Work out the finished part from the listing and answer in its coordinate system (mm). Face numbers are marked on the shaded views. A direction names the side the tool comes from. Round coordinates to 2 decimals unless told otherwise and drop trailing zeros. Write each loop counter-clockwise with the first axis right and the second up, starting at its lowest first coordinate (ties: lowest second). Pieces come first, ordered by that corner, then holes. Notation, with made-up numbers: (39.25, -30.5) - (52.25, -30.5) arc R21 ccw to (52.25, -17.5) - close; hole circle Ø8 at (75, -6.75). An arc over 180 degrees is marked (long way). Write item = value, one per line. Start each with the question number.
Autodesk Inventor part; units mm, degrees
ref_plane "Work Plane1" through (127.7, -30, -88) normal (0, 0, -1) x (-1, 0, 0)
ref_plane "YZ Plane" through (0, 0, 0) normal (1, 0, 0) x (0, 1, 0)
ref_plane "XZ Plane" through (0, 0, 0) normal (0, 1, 0) x (-1, 0, 0)
sketch "Sketch1" plane through (0, 0, 0) normal (0, 0, 1) x (1, 0, 0)
  line L0 (-36, 36) -> (36, 36)
  line L1 (36, 36) -> (36, -36)
  line L2 (36, -36) -> (-36, -36)
  line L3 (-36, -36) -> (-36, 36)
  point P0 (0, 0)
  dimension "d0" = 72
  dimension "d1" = 36
  dimension "d2" = 72
  dimension "d3" = 36
extrude "Plate1" add sketch "Sketch1" along normal blind 6
sketch "Sketch2" plane through (-36, -30, 6) normal (0, -1, 0) x (1, 0, 0)
  line L0 (72, 0) -> (0, 0)
  line L1 (0, 0) -> (0, -94)
  line L2 (0, -94) -> (72, -94)
  line L3 (72, -94) -> (72, 0)
edge flange "Flange1" height 94 angle 90 thickness 6 bend radius 6 thickness toward (0, -1, 0) relief tear relief width 6 relief depth 3 edges at (0, -36, 0) wall of the first edge with corners at (36, -30, 6) (-36, -30, 6) (-36, -30, -88) (36, -30, -88)
bend "Bend1"
corner "Corner1"
sketch "Sketch3" plane through (-36, -30, -88) normal (0, 1, 0) x (1, 0, 0)
  line L0 (72, -82) -> (72, 0)
  line L1 (72, 0) -> (175.7, 0)
  line L2 (175.7, 0) -> (175.7, -60)
  line L3 (175.7, -60) -> (72, -60)
  line L4 (72, -60) -> (72, 0)
  point P0 (36, -88)
  dimension "d15" = 103.7
  dimension "d16" = 60
sheet face with bend "Face2" sketch "Sketch3" thickness 6 toward (0, -1, 0) bend radius 6
bend "Bend2"
sketch "Sketch4" plane through (133.7, -36, -88) normal (1, 0, 0) x (0, 1, 0)
  line L0 (0, 60) -> (0, 0)
  line L1 (0, 0) -> (100.6, 0)
  line L2 (100.6, 0) -> (100.6, 60)
  line L3 (100.6, 60) -> (0, 60)
edge flange "Flange2" height 100.6 angle 90 thickness 6 bend radius 6 thickness toward (1, 0, 0) relief tear relief width 6 relief depth 3 edges at (139.7, -30, -58) wall of the first edge with corners at (133.7, -36, -28) (133.7, -36, -88) (133.7, 64.6, -88) (133.7, 64.6, -28)
bend "Bend3"
corner "Corner2"
sketch "Sketch5" plane through (139.7, 64.6, -28) normal (1, 0, 0) x (0, 0, -1)
  circle A0 centre (30, -30) radius 25
  line L0 (60, 0) -> (60, -88.6)
  line L1 (0, -88.6) -> (0, 0)
  line L2 (0, 0) -> (60, 0)
  point P0 (-28, -64.6)
  point P1 (55, -30)
  point P2 (5, -30)
  dimension "d32" = 60
  dimension "d33" = 30
  dimension "d34" = 30
  dimension "d35" = 50
  dimension "d36" = 30
  dimension "d37" = 30
hole "Hole1" at (139.7, 34.6, -33) at (139.7, 34.6, -83) direction (-1, 0, 0) diameter 5 end through all
sketch "Sketch6" plane through (0, 0, 6) normal (0, 0, 1) x (1, 0, 0)
  circle A0 centre (0, 0) radius 12.7
  line L0 (36, -36) -> (-36, -36)
  circle A1 centre (0, 0) radius 33.5
  line L1 (0, 0) -> (29.0119, -16.75)
  line L2 (0, 0) -> (-29.0119, -16.75)
  line L3 (0, 0) -> (0, 33.5)
  point P0 (0, 0)
  point P1 (0, 12.7)
  point P2 (10.9985, -6.35)
  point P3 (-10.9985, -6.35)
  dimension "d45" = 36
  dimension "d46" = 25.4
  dimension "d47" = 67
  dimension "d48" = 120
  dimension "d49" = 120
  dimension "d50" = 0
hole "Hole2" at (0, 12.7, 6) at (-10.9985, -6.35, 6) at (10.9985, -6.35, 6) at (29.0119, -16.75, 6) at (-29.0119, -16.75, 6) direction (0, 0, -1) diameter 5 end through all
sketch "Sketch7" plane through (-36, -30, -6) normal (0, 1, 0) x (1, 0, 0)
  line L0 (163.7, 82) -> (0, 82)
  line L1 (163.7, 22) -> (72, 22)
  line L2 (0, 0) -> (0, 82)
  line L3 (72, 0) -> (72, 22)
  point P0 (36, -6)
  point P1 (117.85, 52)
  point P2 (36, 52)
  point P3 (36, 11)
  dimension "d65" = 60
  dimension "d66" = 72
  dimension "d67" = 30
  dimension "d68" = 30
  dimension "d69" = 36
  dimension "d70" = 22
  dimension "d71" = 11
  dimension "d72" = 36
  dimension "d73" = 91.7
  dimension "d74" = 45.85
hole "Hole3" at (81.85, -30, -58) at (0, -30, -58) at (0, -30, -17) direction (0, -1, 0) diameter 5 end through all
mirror "Mirror1" about plane through (133.7, -24, -88) normal (0, 0, -1)
ref_plane "Work Plane1" through (127.7, -30, -88) normal (0, 0, -1) x (-1, 0, 0)
split "Split1" plane through (127.7, -30, -88) removes the side toward (0, 0, 1)
equation "\"d2\" = d0"
equation "\"d33\" = 0.5 * d32"
equation "\"d34\" = d33"
equation "\"d36\" = d34"
equation "\"d37\" = d36"
equation "\"d43\" = Thickness"
equation "\"d49\" = d48"
equation "\"d56\" = Thickness"
equation "\"d63\" = Thickness"
equation "\"d4\" = Thickness"
equation "\"d5\" = BendReliefWidth"
equation "\"d6\" = BendReliefDepth"
equation "\"d7\" = MinimumRemnant"
equation "\"d8\" = TransitionRadius"
equation "\"d11\" = BendRadius"
equation "\"d12\" = CornerReliefSize"
equation "\"d13\" = GapSize"
equation "\"d14\" = JacobiRadiusSize"
equation "\"d17\" = BendRadius"
equation "\"d18\" = BendReliefWidth"
equation "\"d20\" = MinimumRemnant"
equation "\"d19\" = BendReliefDepth"
equation "\"d21\" = TransitionRadius"
equation "\"d22\" = BendReliefWidth"
equation "\"d23\" = BendReliefDepth"
equation "\"d24\" = MinimumRemnant"
equation "\"d25\" = TransitionRadius"
equation "\"d28\" = BendRadius"
equation "\"d29\" = CornerReliefSize"
equation "\"d30\" = GapSize"
equation "\"d31\" = JacobiRadiusSize"
equation "\"BendRadius\" = Thickness"
equation "\"BendReliefWidth\" = Thickness"
equation "\"BendReliefDepth\" = 0.5 * Thickness"
equation "\"CornerReliefSize\" = 4 * Thickness"
equation "\"MinimumRemnant\" = 2 * Thickness"
equation "\"TransitionRadius\" = BendRadius"
equation "\"JacobiRadiusSize\" = BendRadius"
equation "\"GapSize\" = Thickness"
properties part number "motorHolder_flipped"
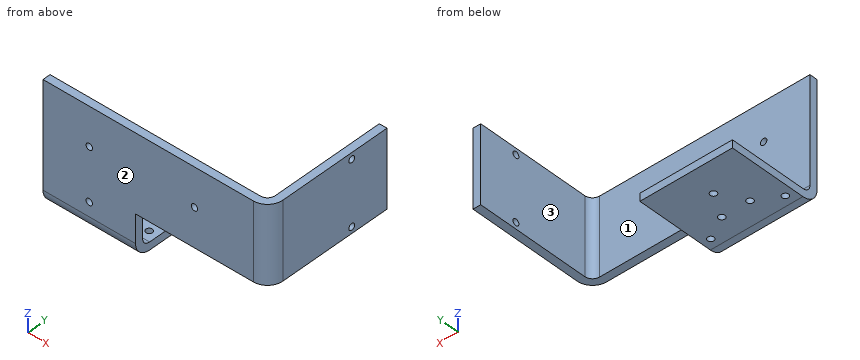
1. Which of the six approach directions +Z, -Z, +X, -X, +Y, -Y give full straight-line access (tool end or side, diameter ignored) to the marked faces 1, 2 and 3?
2. Find section B-B on z = -93. Give the vertices of the cut face in (x, y).
3. Find section C-C on y = 27.5. Give the vertices of the cut face in (x, z), plus the area to 3 significant figures.
4. Find section A-A on x = 81.85. Give the vertices of the cut face in (y, z).
5. Each of these flat-tipped pins is pushed along its axis until it touches: pin 1 (12 mm diameter, centred on x = 51.5, y = -20.5, fed in from -Z); pin 2 (6.5 mm diameter, centred on x = -29.01, y = -16.75, fed in from -Z); pin 3 (8 mm diameter, centred on y = 34.6, z = -93, fed in from -X); pin 4 (1.5 mm diameter, centred on x = 32, y = -13.5, fed in from +Z). Where does it stop, or does it pass through?
6. Consider line 1 (Z direction, x = 136.95, y = 34.6); line 2 (X direction, y = -6.35, z = -179.3); line 3 (X direction, y = 12.5, z = -176.5). Determine where each line is inside the solid, lowest interval first.
7. Find section D-D on x = 0. Give the vertices of the cut face in (y, z), plus the area to 3 significant figures.
Answer key:
q1.face_1 = +Z, -X, +Y
q1.face_2 = +Z, -Z, +X, -X, -Y
q1.face_3 = +Z, -Z, -X, +Y
q2.outline = (-36, -36) - (127.7, -36) arc R12 ccw to (139.7, -24) - (139.7, 32.1) - (133.7, 32.1) - (133.7, -24) arc R6 cw to (127.7, -30) - (-36, -30) - close; (133.7, 37.1) - (139.7, 37.1) - (139.7, 64.6) - (133.7, 64.6) - close
q3.outline = (-36, -182) - (36, -182) - (36, -176) - (-36, -176) - close; (133.7, -148) - (139.7, -148) - (139.7, -88) - (133.7, -88) - close
q3.area = 792 mm²
q4.outline = (-36, -148) - (-30, -148) - (-30, -120.5) - (-36, -120.5) - close; (-36, -115.5) - (-30, -115.5) - (-30, -88) - (-36, -88) - close
q5.pin_1 = through
q5.pin_2 = -182
q5.pin_3 = 133.7
q5.pin_4 = -176
q6.line_1 = -148 to -145.5, -140.5 to -95.5, -90.5 to -88
q6.line_2 = -36 to -13.5, -8.5 to 8.5, 13.5 to 36
q6.line_3 = -36 to -2.49, 2.49 to 36
q7.outline = (-36, -170) arc R12 ccw to (-24, -182) - (10.2, -182) - (10.2, -176) - (-24, -176) arc R6 cw to (-30, -170) - (-30, -161.5) - (-36, -161.5) - close; (-36, -156.5) - (-30, -156.5) - (-30, -120.5) - (-36, -120.5) - close; (-36, -115.5) - (-30, -115.5) - (-30, -88) - (-36, -88) - close; (15.2, -182) - (36, -182) - (36, -176) - (15.2, -176) - close
q7.area = 847 mm²
